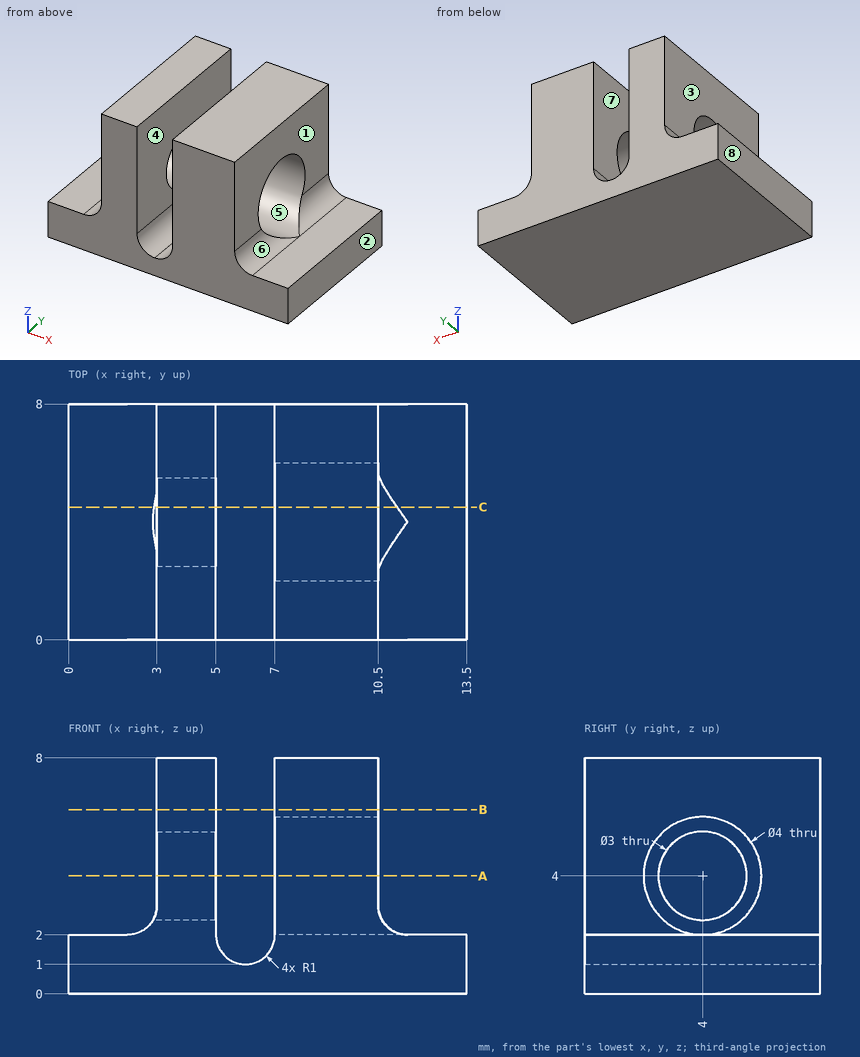
The figure shows three views and two pictorial views of one solid part (mm, origin at its lowest corner). Answer the questions. A direction names the side the tool comes from. Round coordinates to 2 decimals unless told otherwise and drop trailing zeros. Write each loop counter-clockwise with the first axis right and the second up, starting at its lowest first coordinate (ties: lowest second). Pieces come first, ordered by that corner, then holes. Notation, with made-up numbers: (80, -26) - (115, -26) arc R18 ccw to (115, -7) - close; hole circle Ø10 at (-10, 67). An arc over 180 degrees is marked (long way). Use one line per item in the form item = value. Start each with the question number.
Item 1: Find the intervals of material crossed by line 1 (X direction, y = 7, z = 4.25); line 2 (Y direction, x = 8.2, z = 4); line 3 (Y direction, x = 4.5, z = 4), in increasing order. Write a range as [from, to].
Item 2: A cutting plane is placed at B-B (z = 6.25). Write down the section's boundary in (x, y), plus the area to 3 significant figures.
Item 3: Determine the mould class of the marked faces 6, 7 and 8 for opening direction X: +X half, -X half, draft (parallel to the pull), parting line (faces both ways), or undercut.
Item 4: A cutting plane is placed at A-A (z = 4). Write down the section's boundary in (x, y).
Item 5: Flat-ended cylindrical pins translate along their axes: pin 1 Ø3 at (y, z) = (3, 5) entering from -X; pin 2 Ø1.6 at (x, y) = (1.5, 5.5) entering from +Z (1 decimal). Find the tip coordinate at first contact, or state that the pin passes through.
Item 6: A cutting plane is placed at C-C (y = 4.5). Give the number of separate pieces and of enclosed holes in the cut face.
Item 7: A tool of negligible diameter and unlimited length cuts with its end or side. For the marked faces 1, 2, 3, 4 and 5, from which of +Z, -Z, +X, -X, +Y, -Y can it reach the whole face along a straight path? Write none if from no direction.
The answers:
q1.line_1 = [3, 5], [7, 10.5]
q1.line_2 = [0, 2], [6, 8]
q1.line_3 = [0, 2.5], [5.5, 8]
q2.outline = (3, 0) - (5, 0) - (5, 8) - (3, 8) - close; (7, 0) - (10.5, 0) - (10.5, 8) - (7, 8) - close
q2.area = 44.0 mm^2
q3.face_6 = +X half
q3.face_7 = undercut
q3.face_8 = -X half
q4.outline = (3, 0) - (5, 0) - (5, 2.5) - (3, 2.5) - close; (3, 5.5) - (5, 5.5) - (5, 8) - (3, 8) - close; (7, 0) - (10.5, 0) - (10.5, 2) - (7, 2) - close; (7, 6) - (10.5, 6) - (10.5, 8) - (7, 8) - close
q5.pin_1 = 3
q5.pin_2 = 2
q6.separate_pieces = 3
q6.enclosed_holes = 0
q7.face_1 = +Z, +X, +Y, -Y
q7.face_2 = +Z, -Z, +X, +Y, -Y
q7.face_3 = +Z, -X, +Y, -Y
q7.face_4 = +Z, +Y, -Y
q7.face_5 = +X
